```python
from build123d import *

# Parameters (mm, degrees)
BOSS_EXTRUDE1_DEPTH     = 10.8
BOSS_EXTRUDE2_DEPTH     = 10.64
CUT_EXTRUDE1_DEPTH      = 39.168054705
CUT_EXTRUDE1_DEPTH_BACK = 39.168054705
SKETCH5_R               = 5
FILLET1_R               = 1
SKETCH6_W               = 21.28
SKETCH6_H               = 16.18
BOSS_EXTRUDE3_DEPTH     = 12
SKETCH7_W               = 5
SKETCH7_H               = 21.281328743
BOSS_EXTRUDE4_DEPTH     = 56.83
SKETCH8_W               = 21.284331222
SKETCH8_H               = 16.18
BOSS_EXTRUDE5_DEPTH     = 7.19
FILLET3_R               = 3
SKETCH9_R               = 2.2
CUT_EXTRUDE2_DEPTH      = 85.918196519
SKETCH10_R              = 3.175
CUT_EXTRUDE3_DEPTH      = 85.918196519
SKETCH11_W              = 24.977296572
SKETCH11_H              = 9.721484234
CUT_EXTRUDE4_DEPTH      = 71.220021919
CUT_EXTRUDE6_DEPTH      = 90.46728118


with BuildPart() as part:
    # Sketch2 → Boss-Extrude1 (new body)
    with BuildSketch(Plane.XY):
        Polygon((-10.1, 0), (0, 0), (0, 7), (-6.25480432, 7), (-10.1, 1.709943763), align=None)
        Polygon((0, 0), (10.1, 0), (10.1, 1.709943763), (6.25480432, 7), (0, 7), align=None)
    extrude(amount=BOSS_EXTRUDE1_DEPTH)

    # Sketch4 → Boss-Extrude2 (add, symmetric)
    with BuildSketch(Plane.XY):
        Polygon((-4, 0), (-4, -4.8), (-30, -4.8), (-30, -20.98), (30, -20.98), (30, -4.8), (4, -4.8), (4, 0), align=None)
    extrude(amount=BOSS_EXTRUDE2_DEPTH, both=True)

    # Sketch5 → Cut-Extrude1 (cut, two sides: drawn at the far end of the back side and taken through both)
    with BuildSketch(Plane.XY.offset(-CUT_EXTRUDE1_DEPTH_BACK)):
        with Locations((-22.790976064, -22.227391232)):
            Circle(SKETCH5_R)
        with Locations((22.790976064, -22.227391232)):
            Circle(SKETCH5_R)
    extrude(amount=CUT_EXTRUDE1_DEPTH + CUT_EXTRUDE1_DEPTH_BACK, mode=Mode.SUBTRACT)

    # Fillet1
    fillet1_edges = [part.edges().sort_by_distance(p)[0] for p in [
        (-10.1, 0, 5.4),
        (-10.1, 1.709943763, 5.4),
        (-6.25480432, 7, 5.4),
        (6.25480432, 7, 5.4),
        (10.1, 1.709943763, 5.4),
        (10.1, 0, 5.4),
    ]]
    fillet(fillet1_edges, radius=FILLET1_R)

    # Sketch6 → Boss-Extrude3 (add)
    with BuildSketch(Plane(origin=(30, 0, 0), x_dir=(0, 0, -1), z_dir=(1, 0, 0))):
        with Locations((0, -12.89)):
            Rectangle(SKETCH6_W, SKETCH6_H)
    extrude(amount=BOSS_EXTRUDE3_DEPTH)

    # Sketch7 → Boss-Extrude4 (add)
    with BuildSketch(Plane(origin=(0, -4.8, 0), x_dir=(1, 0, 0), z_dir=(0, 1, 0))):
        with Locations((39.5, 0.000664372)):
            Rectangle(SKETCH7_W, SKETCH7_H)
    extrude(amount=BOSS_EXTRUDE4_DEPTH)

    # Sketch8 → Boss-Extrude5 (add)
    with BuildSketch(Plane.ZY.offset(-37)):
        with Locations((0.000836868, 43.94)):
            Rectangle(SKETCH8_W, SKETCH8_H)
    extrude(amount=BOSS_EXTRUDE5_DEPTH)

    # Fillet3
    fillet3_edges = [part.edges().sort_by_distance(p)[0] for p in [
        (42, -20.98, 0),
        (42, 52.03, -0.000664372),
    ]]
    fillet(fillet3_edges, radius=FILLET3_R)

    # Sketch9 → Cut-Extrude2 (cut, through all)
    with BuildSketch(Plane.XZ.offset(20.98)):
        with Locations((32.632878078, 0)):
            Circle(SKETCH9_R)
    extrude(amount=-CUT_EXTRUDE2_DEPTH, mode=Mode.SUBTRACT)

    # Sketch10 → Cut-Extrude3 (cut, through all)
    with BuildSketch(Plane.XZ.offset(20.98)):
        with Locations((0.000925951, 0)):
            Circle(SKETCH10_R)
    extrude(amount=-CUT_EXTRUDE3_DEPTH, mode=Mode.SUBTRACT)

    # Sketch11 → Cut-Extrude4 (cut, through all)
    with BuildSketch(Plane.XY.offset(10.8)):
        with Locations((-0.121132817, 4.060742117)):
            Rectangle(SKETCH11_W, SKETCH11_H)
    extrude(amount=-CUT_EXTRUDE4_DEPTH, mode=Mode.SUBTRACT)

    # Sketch13 → Cut-Extrude6 (cut, through all)
    with BuildSketch(Plane(origin=(42, 0, 0), x_dir=(0, 0, -1), z_dir=(1, 0, 0))):
        with BuildLine():
            Line((3.175, 21.525), (3.175, 9.525))
            ThreePointArc((3.175, 9.525), (0, 6.35), (-3.175, 9.525))
            Line((-3.175, 9.525), (-3.175, 21.525))
            ThreePointArc((-3.175, 21.525), (0, 24.7), (3.175, 21.525))
        make_face()
    extrude(amount=-CUT_EXTRUDE6_DEPTH, mode=Mode.SUBTRACT)


solid = part.part
```
Design review of the part built by this model. Coordinates are the model's own, in mm. A direction names the side the tool comes from. Give positions to 0.01 mm unless a question says otherwise; leave off trailing zeros. Write each loop counter-clockwise with the first axis right and the second up, starting at its lowest first coordinate (ties: lowest second). Pieces come first, ordered by that corner, then holes.
(1) Mouldability with a two-part tool opening along X and no side actions: class faces 1 (the face through (22.88, -17.23, -0.15)), 2 (the face through (41.14, -20.08, -0.15)), 3 (the face through (-4, -3, 0)), 4 (the face through (35, 35.85, 0)) as +X half, -X half, draft (parallel to the pull), parting line (faces both ways), or undercut.
Checked values:
face 1: undercut
face 2: +X half
face 3: -X half
face 4: draft
(2) Add section A-A (z = 0). Give the number of separate pieces and of enclosed holes in the cut face, and give its area (3 significant figures).
Checked values:
separate pieces: 5
enclosed holes: 0
area: 1,180 mm2
(3) Wall thickness on line 1 along Y through (x, z) = (35.5, 9); line 2 along X through (y, z) = (-16, -1.25); line 3 along Y through (x, z) = (-16, -0.5): over which ranges is each line inside the solid? List them lowest first.
Checked values:
line 1: y = -20.98 to -4.8, 35.85 to 52.03
line 2: x = -30 to -2.92, 2.92 to 30.82, 34.44 to 42
line 3: y = -20.98 to -4.8
(4) Clearance check with flat-ended pins moving along their axes: pin 1 Ø9 at (x, z) = (1.5, -2.5) entering from +Y; pin 2 Ø10.5 at (y, z) = (17, -1.5) entering from -X; pin 3 Ø4 at (x, z) = (-9, -1.5) entering from +Y; pin 4 Ø3 at (x, y) = (33.5, -4) entering from -Z. State where each tip first meets the part, or that it passes through.
Checked values:
pin 1: stops at y = -0.8
pin 2: stops at x = 37
pin 3: stops at y = -4.8
pin 4: stops at z = -10.64
(5) Add section C-C (y = -11.5). Give the boundary of the cut face in (x, z) (3 decimals), and give its area (3 significant figures).
Checked values:
outline: (-30, -10.64) - (42, -10.64) - (42, 10.64) - (-30, 10.64) - close; hole circle Ø6.35 at (0.001, 0); hole circle Ø4.4 at (32.633, 0)
area: 1,490 mm2
(6) Tool access review of faces 5 (the face through (-22.7, -17.23, -0.15)), 6 (the face through (20, -4.8, 0)), 7 (the face through (40, 15, 3.175)), 8 (the face through (42, 15, 5)), 9 (the face through (-17, -4.8, 0)): name each direction out of +Z, -Z, +X, -X, +Y, -Y from which nothing blocks a thin tool from reaching the whole face with its end or side.
Checked values:
face 5: +Z, -Z, -Y
face 6: +Z, -Z
face 7: +X, -X
face 8: +Z, -Z, +X, +Y, -Y
face 9: +Z, -Z, -X, +Y
(7) Add section B-B (x = 0). Give the boundary of the cut face in (y, z) (3 decimals).
Checked values:
outline: (-20.98, -10.64) - (-0.8, -10.64) - (-0.8, -3.175) - (-20.98, -3.175) - close; (-20.98, 3.175) - (-0.8, 3.175) - (-0.8, 10.64) - (-20.98, 10.64) - close
(8) Add section D-D (z = 4.5). Give the boundary of the cut face in (x, y), and give its area (3 significant figures).
Checked values:
outline: (-30, -20.98) - (-27.63, -20.98) arc R5 cw to (-17.95, -20.98) - (17.95, -20.98) arc R5 cw to (27.63, -20.98) - (39, -20.98) arc R3 ccw to (42, -17.98) - (42, 49.03) arc R3 ccw to (39, 52.03) - (29.81, 52.03) - (29.81, 35.85) - (37, 35.85) - (37, -4.8) - (4, -4.8) - (4, -0.8) - (-4, -0.8) - (-4, -4.8) - (-30, -4.8) - close
area: 1,540 mm2
